```python
from build123d import *

# Parameters (mm, degrees)
SKETCH1_W          = 76.2
SKETCH1_H          = 35.2
BASE_SHAPE_DEPTH   = 2.7
SKETCH2_R          = 6
SKETCH2_R_2        = 1.75
MOTOR_HOLES_DEPTH  = 43.055439601
SKETCH3_W          = 12.7
SKETCH3_H          = 2.7
TOP_TEETH_DEPTH    = 5.334
SKETCH4_W          = 12.7
SKETCH4_H          = 2.7
BOTTOM_TEETH_DEPTH = 5.334


with BuildPart() as part:
    # Sketch1 → Base Shape (new body)
    with BuildSketch(Plane.XY):
        Rectangle(SKETCH1_W, SKETCH1_H)
    extrude(amount=-BASE_SHAPE_DEPTH)

    # Sketch2 → Motor Holes (cut, through all)
    with BuildSketch(Plane.XY):
        with Locations((0, -8.73)):
            Circle(SKETCH2_R)
        with Locations((-10.25, -8.73)):
            Circle(SKETCH2_R_2)
        with Locations((10.25, -8.73)):
            Circle(SKETCH2_R_2)
        with Locations((0, 13.369999996)):
            Circle(SKETCH2_R_2)
    extrude(amount=-MOTOR_HOLES_DEPTH, mode=Mode.SUBTRACT)

    # Sketch3 → Top teeth (add)
    with BuildSketch(Plane(origin=(0, 17.6, 0), x_dir=(1, 0, 0), z_dir=(0, 1, 0))):
        with Locations((-31.75, 1.35)):
            Rectangle(SKETCH3_W, SKETCH3_H)
        with Locations((0, 1.35)):
            Rectangle(SKETCH3_W, SKETCH3_H)
        with Locations((31.75, 1.35)):
            Rectangle(SKETCH3_W, SKETCH3_H)
    extrude(amount=TOP_TEETH_DEPTH)

    # Sketch4 → Bottom teeth (add)
    with BuildSketch(Plane.XZ.offset(17.6)):
        with Locations((-31.75, -1.35)):
            Rectangle(SKETCH4_W, SKETCH4_H)
        with Locations((0, -1.35)):
            Rectangle(SKETCH4_W, SKETCH4_H)
        with Locations((31.75, -1.35)):
            Rectangle(SKETCH4_W, SKETCH4_H)
    extrude(amount=BOTTOM_TEETH_DEPTH)


solid = part.part
```
Part model, mm, in its own coordinate system. A direction names the side the tool comes from. Round coordinates to 2 decimals unless told otherwise and drop trailing zeros. Order: outer loops, then holes, each group sorted by start corner. A loop starts at its lowest first (then second) coordinate and runs counter-clockwise, first axis right, second up. Notation, with made-up numbers: M -39,34 L -19,34 A10 ccw -19,44 Z; hole C -6,15.25 d6. An arc over 180 degrees is marked long. Answer in a Markdown table with one row per item. Add a question column.
Q1. Cut at C-C on z = -1.9. Give the cut face in (x, y), and give its area (3 significant figures).
Q2. Cut at B-B on x = 0. Give the cut face in (y, z), and give its area (3 significant figures).
Q3. Cut at A-A on x = 10.25. Give the cut face in (y, z), and give its area (3 significant figures).
Q4. Mould opens along Y. For faces 4 (the face through (-8.633, -9.4, -1.331)), 5 (the face through (16, 17.6, -1)), 6 (the face through (32, -22.934, -1)), 7 (the face through (-38.1, 0, -1)) say: +Y half, -Y half, draft (parallel to the pull), parting line (faces both ways), or undercut.
Q5. Wall check: L1, parallel to Y at x = 0, z = -0.85; L2, parallel to X at y = 13.37, z = -2.1; L3, parallel to X at y = -5.5, z = -2.2. Give the ranges that are in metal, low to high. Write a range as from..to.
Q6. Cut at D-D on y = -8.73. Give the cut face in (x, z).
Q7. 3-axis set-ups, long thin cutter, end or side, ignore diameter. For faces 1 (the face through (25.4, 20, -1)), 2 (the face through (-16, -17.6, -1)), 3 (the face through (-1, 0, 0)): which of +Z, -Z, +X, -X, +Y, -Y reach the whole face in a straight line?
Q8. Pin check, flat tip, straight feed: pin 1 (9.5 mm diameter, centred on x = 0, y = -8.73, fed in from -Z). Stop position of the tip, or through.
Established:
| question | item | result |
|---|---|---|
| 1 | outline | M -38.1,-22.93 L -25.4,-22.93 L -25.4,-17.6 L -6.35,-17.6 L -6.35,-22.93 L 6.35,-22.93 L 6.35,-17.6 L 25.4,-17.6 L 25.4,-22.93 L 38.1,-22.93 L 38.1,22.93 L 25.4,22.93 L 25.4,17.6 L 6.35,17.6 L 6.35,22.93 L -6.35,22.93 L -6.35,17.6 L -25.4,17.6 L -25.4,22.93 L -38.1,22.93 Z; hole C -10.25,-8.73 d3.5; hole C 0,-8.73 d12; hole C 0,13.37 d3.5; hole C 10.25,-8.73 d3.5 |
| 1 | area | 2,950 mm2 |
| 2 | outline | M -22.93,-2.7 L -14.73,-2.7 L -14.73,0 L -22.93,0 Z; M -2.73,-2.7 L 11.62,-2.7 L 11.62,0 L -2.73,0 Z; M 15.12,-2.7 L 22.93,-2.7 L 22.93,0 L 15.12,0 Z |
| 2 | area | 82.0 mm2 |
| 3 | outline | M -17.6,-2.7 L -10.48,-2.7 L -10.48,0 L -17.6,0 Z; M -6.98,-2.7 L 17.6,-2.7 L 17.6,0 L -6.98,0 Z |
| 3 | area | 85.6 mm2 |
| 4 | face 4 | undercut |
| 4 | face 5 | +Y half |
| 4 | face 6 | -Y half |
| 4 | face 7 | draft |
| 5 | L1 | y = -22.93..-14.73, -2.73..11.62, 15.12..22.93 |
| 5 | L2 | x = -38.1..-1.75, 1.75..38.1 |
| 5 | L3 | x = -38.1..-5.06, 5.06..38.1 |
| 6 | outline | M -38.1,-2.7 L -12,-2.7 L -12,0 L -38.1,0 Z; M -8.5,-2.7 L -6,-2.7 L -6,0 L -8.5,0 Z; M 6,-2.7 L 8.5,-2.7 L 8.5,0 L 6,0 Z; M 12,-2.7 L 38.1,-2.7 L 38.1,0 L 12,0 Z |
| 7 | face 1 | +Z, -Z, +Y |
| 7 | face 2 | +Z, -Z, -Y |
| 7 | face 3 | +Z, +X, -X, +Y, -Y |
| 8 | pin 1 | passes through |
